The model under review builds one solid part; all positions refer to its coordinate system, in mm. A direction names the side the tool comes from. Give positions to 0.01 mm unless a question says otherwise; leave off trailing zeros. Order: outer loops, then holes, each group sorted by start corner. A loop starts at its lowest first (then second) coordinate and runs counter-clockwise, first axis right, second up. Notation, with made-up numbers: M 16.5,50.5 L 40.5,50.5 A12 ccw 40.5,66.5 Z; hole C 31,10.5 d4. An arc over 180 degrees is marked long. One line per question, with ' | ' between items. Start each with the question number.
1. We need section D-D on z = 6.5. Write out the cut boundary in (x, y), then the cut area to 3 significant figures.
2. Wall thickness on L1, parallel to Y at x = 0, z = 14.5; L2, parallel to Y at x = -1.5, z = -14; L3, parallel to X at y = 1.25, z = 14.5: over which ranges is each line inside the solid? List them lowest first.
3. We need section C-C on z = -15.5. Write out the cut boundary in (x, y).
4. For faces 1 (the face through (-5, 0, 25.4)), 2 (the face through (5.158, -3.955, 11.795)), 3 (the face through (5.158, -3.955, 23.893)), list the 3-axis set-ups (+Z, -Z, +X, -X, +Y, -Y) from which the entire face can be reached by the end or side of a thin tool; tool diameter is ignored.
5. Insertion check: P1, Ø2, axis at x = -3, y = 1.5, coming from the -Z side; P2, Ø1, axis at y = 0.5, z = 19.5, coming from the -X side; P3, Ø4, axis at x = 2.5, z = -8.5, coming from the -Y side; P4, Ø1, axis at x = 6, z = 8.5, coming from the +Y side. Each pin has a flat end and moves straight along its axis. Give the tip position at first contact, or say it passes through.
6. The part is to be moulded in two halves that separate along Z. For faces 4 (the face through (1.73, -7.81, -4.2)), 5 (the face through (4.9, 4.5, 4.3)), 6 (the face through (0, -5, -19)), say which applies: +Z half, -Z half, draft (parallel to the pull), parting line (faces both ways), or undercut.
7. We need section A-A on y = 0. Write out the cut boundary in (x, z), then the cut area to 3 significant figures.
```python
from build123d import *

# Parameters (mm, degrees)
F2_SIZE = 1


with BuildPart() as f1:
    # F0 (on Front) → F1 (revolve)
    with BuildSketch(Plane.XZ):
        Polygon((-4.5, -19), (-4.5, 25.4), (-6.5, 25.4), (-6.5, 23.4), (-7, 21.4), (-6.5, 19.4), (-6.5, 4.4), (-8, 3.4), (-8, -11.6), (-8.5, -14.1), (-8, -16.6), (-7.033584, -19), align=None)
    revolve(axis=Axis((0, 0, -3.23939), (0, 0, -1)))

    # F2
    f2_edges = [f1.edges().sort_by_distance(p)[0] for p in [
        (6.5, 0, 25.4),
    ]]
    chamfer(f2_edges, length=F2_SIZE)


solid = f1.part
```
Entries:
1) outline: C 0,0 d13; hole C 0,0 d9 | area: 69.1 mm^2
2) L1: y = -6.5 to -4.5, 4.5 to 6.5 | L2: y = -8.35 to -4.24, 4.24 to 8.35 | L3: x = -6.38 to -4.32, 4.32 to 6.38
3) outline: C 0,0 d16.44; hole C 0,0 d9
4) face 1: +Z, +X, -X, +Y, -Y | face 2: none | face 3: +Z
5) P1: passes through | P2: stops at x = -6.64 | P3: stops at y = -7.98 | P4: stops at y = 3.46
6) face 4: draft | face 5: undercut | face 6: -Z half
7) outline: M -8.5,-14.1 L -8,-16.6 L -7.03,-19 L -4.5,-19 L -4.5,25.4 L -5.5,25.4 L -6.5,24.4 L -6.5,23.4 L -7,21.4 L -6.5,19.4 L -6.5,4.4 L -8,3.4 L -8,-11.6 Z; M 4.5,-19 L 7.03,-19 L 8,-16.6 L 8.5,-14.1 L 8,-11.6 L 8,3.4 L 6.5,4.4 L 6.5,19.4 L 7,21.4 L 6.5,23.4 L 6.5,24.4 L 5.5,25.4 L 4.5,25.4 Z | area: 247 mm^2
